Build history of the part. All positions in model axes, mm. A direction names the side the tool comes from. Round coordinates to 2 decimals unless told otherwise and drop trailing zeros. Write each loop counter-clockwise with the first axis right and the second up, starting at its lowest first coordinate (ties: lowest second). Pieces come first, ordered by that corner, then holes.
Item 1: Wall check: probe 1 along X at (y, z) = (9.5, 1.5); probe 2 along X at (y, z) = (4.75, 0.85); probe 3 along Y at (x, z) = (-6.5, 1.2). Give the ranges that are in metal, low to high.
Item 2: Band-saw the part on A-A, the plane z = 1.5. Write the cut outline in (x, y), then the cut area to 3 significant figures.
Item 3: 3-axis set-ups, long thin cutter, end or side, ignore diameter. For faces 5 (the flat face through (-6.35, 3, 2)), 6 (the flat face through (0, -1, 3)), 7 (the cylindrical face through (10.33, 8.62, 1.7)): which of +Z, -Z, +X, -X, +Y, -Y reach the whole face in a straight line?
Item 4: Drop flat-ended pins along their axis: pin 1 Ø0.9 at (x, z) = (2.5, 1.5) entering from +Y; pin 2 Ø4 at (x, y) = (-5, 3.5) entering from -Z. Give the stop position or say it passes through.
Item 5: Band-saw the part on C-C, the plane y = 10. Write the cut outline in (x, z) (3 decimals), then the cut area to 3 significant figures.
Item 6: Band-saw the part on B-B, the plane x = -4.25. Write the cut outline in (y, z).
Item 7: Mould opens along X. For faces 1 (the flat face through (-12.5, 0, 1)), 2 (the flat face through (12.5, 0, 1)), 3 (the flat face through (0, -6.25, 1)), 4 (the flat face through (8.7, 6.25, 0.5)) say: +X half, -X half, draft (parallel to the pull), parting line (faces both ways), or undercut.
```python
from build123d import *

# Parameters (mm, degrees)
SKETCH1_W           = 25
SKETCH1_H           = 12.5
BOSS_EXTRUDE1_DEPTH = 3
SKETCH2_W           = 12.7
SKETCH2_H           = 6.35
CUT_EXTRUDE1_DEPTH  = 3
SKETCH3_R           = 0.925
BOSS_EXTRUDE2_DEPTH = 4.8


with BuildPart() as part:
    # Sketch1 → Boss-Extrude1 (new body)
    with BuildSketch(Plane.XY):
        Rectangle(SKETCH1_W, SKETCH1_H)
    extrude(amount=BOSS_EXTRUDE1_DEPTH)

    # Sketch2 → Cut-Extrude1 (cut)
    with BuildSketch(Plane.XY.offset(3)):
        with Locations((0, 3.075)):
            Rectangle(SKETCH2_W, SKETCH2_H)
    extrude(amount=-CUT_EXTRUDE1_DEPTH, mode=Mode.SUBTRACT)

    # Sketch3 → Boss-Extrude2 (add)
    with BuildSketch(Plane(origin=(0, 6.25, 0), x_dir=(1, 0, 0), z_dir=(0, 1, 0))):
        with Locations(Location((-9.425, -1.5, 0), (0, 0, 90))):
            Circle(SKETCH3_R)
        with Locations(Location((9.425, -1.5, 0), (0, 0, 90))):
            Circle(SKETCH3_R)
    extrude(amount=BOSS_EXTRUDE2_DEPTH)


solid = part.part
```
Results:
1. probe 1: x = -10.35 to -8.5, 8.5 to 10.35
1. probe 2: x = -12.5 to -6.35, 6.35 to 12.5
1. probe 3: y = -6.25 to 6.25
2. outline: (-12.5, -6.25) - (12.5, -6.25) - (12.5, 6.25) - (10.35, 6.25) - (10.35, 11.05) - (8.5, 11.05) - (8.5, 6.25) - (6.35, 6.25) - (6.35, -0.1) - (-6.35, -0.1) - (-6.35, 6.25) - (-8.5, 6.25) - (-8.5, 11.05) - (-10.35, 11.05) - (-10.35, 6.25) - (-12.5, 6.25) - close
2. area: 250 mm2
3. face 5: +Z, -Z, +Y
3. face 6: +Z, +X, -X, +Y, -Y
3. face 7: +Y
4. pin 1: stops at y = -0.1
4. pin 2: stops at z = 0
5. outline: circle Ø1.85 at (-9.425, 1.5); circle Ø1.85 at (9.425, 1.5)
5. area: 5.38 mm2
6. outline: (-6.25, 0) - (-0.1, 0) - (-0.1, 3) - (-6.25, 3) - close
7. face 1: -X half
7. face 2: +X half
7. face 3: draft
7. face 4: undercut
